```python
from build123d import *

# Parameters (mm, degrees)
F0_R     = 22.5
F0_R_2   = 12.55
F1_DEPTH = 20
F2_R     = 2.5
F3_R     = 1
F4_R     = 1
F5_R     = 2.5


with BuildPart() as f1:
    # F0 (on Top) → F1 (new body)
    with BuildSketch(Plane.XY):
        Circle(F0_R)
        Circle(F0_R_2, mode=Mode.SUBTRACT)
    extrude(amount=F1_DEPTH)

    # F2
    f2_edges = [f1.edges().sort_by_distance(p)[0] for p in [
        (-22.5, 0, 20),
    ]]
    fillet(f2_edges, radius=F2_R)

    # F3
    f3_edges = [f1.edges().sort_by_distance(p)[0] for p in [
        (-12.55, 0, 20),
    ]]
    fillet(f3_edges, radius=F3_R)

    # F4
    f4_edges = [f1.edges().sort_by_distance(p)[0] for p in [
        (-12.55, 0, 0),
    ]]
    fillet(f4_edges, radius=F4_R)

    # F5
    f5_edges = [f1.edges().sort_by_distance(p)[0] for p in [
        (-22.5, 0, 0),
    ]]
    fillet(f5_edges, radius=F5_R)


solid = f1.part
```
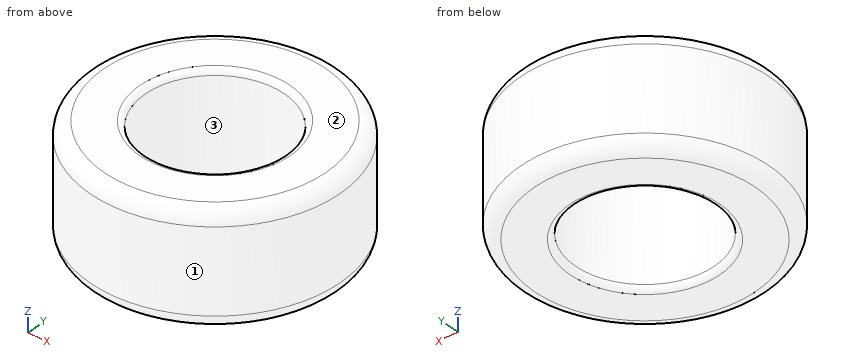
Geometry check sheet. Reference: the model listing, model coordinates, mm. Face numbers are marked on the shaded views. Coordinates: 2 decimals unless noted, no trailing zeros. Write each loop counter-clockwise with the first axis right and the second up, starting at its lowest first coordinate (ties: lowest second). Pieces come first, ordered by that corner, then holes. Notation, with made-up numbers: M 83.5,54.5 L 106.5,54.5 A18 ccw 106.5,84.5 Z; hole C 40,18.25 d11. An arc over 180 degrees is marked long. One line per item, written item: value. Start each with the question number.
(1) Depth check by flat-ended pin: pin 1 (2 mm diameter, centred on x = -17.5, y = 13.5, fed in from -Z); pin 2 (8 mm diameter, centred on x = 6, y = -3.5, fed in from +Z); pin 3 (1.5 mm diameter, centred on y = 5.5, z = 14, fed in from -X); pin 4 (1.5 mm diameter, centred on y = 14.5, z = 12.5, fed in from +X). Enter the tip coordinate at first touch or a pass-through.
(2) Scan lines: line 1 along Y through (x, z) = (0, 5.5); line 2 along X through (y, z) = (-9, 13.5); line 3 along Y through (x, z) = (-10, 11.25). Record each from-to range of solid material in increasing order. Write a range as [from, to].
(3) Sectioned sample at C-C, the plane z = 8. Enter the section's corners in (x, y), and give its area (3 significant figures).
(4) Release check for a two-part mould opening along X. For the marked faces 1, 2 and 3 record: released by +X, released by -X, zero draft, split by the parting line, or undercut.
(5) Sectioned sample at A-A, the plane x = 0. Enter the section's corners in (y, z), and give its area (3 significant figures).
Filled sheet:
1. pin 1: z = 0.26
1. pin 2: through
1. pin 3: x = -21.99
1. pin 4: x = 17.81
2. line 1: [-22.5, -12.55], [12.55, 22.5]
2. line 2: [-20.62, -8.75], [8.75, 20.62]
2. line 3: [-20.16, -7.58], [7.58, 20.16]
3. outline: C 0,0 d45; hole C 0,0 d25.1
3. area: 1,100 mm²
4. face 1: split by the parting line
4. face 2: zero draft
4. face 3: undercut
5. outline: M -22.5,2.5 A2.5 ccw -20,0 L -13.55,0 A1 ccw -12.55,1 L -12.55,19 A1 ccw -13.55,20 L -20,20 A2.5 ccw -22.5,17.5 Z; M 12.55,1 A1 ccw 13.55,0 L 20,0 A2.5 ccw 22.5,2.5 L 22.5,17.5 A2.5 ccw 20,20 L 13.55,20 A1 ccw 12.55,19 Z
5. area: 392 mm²
